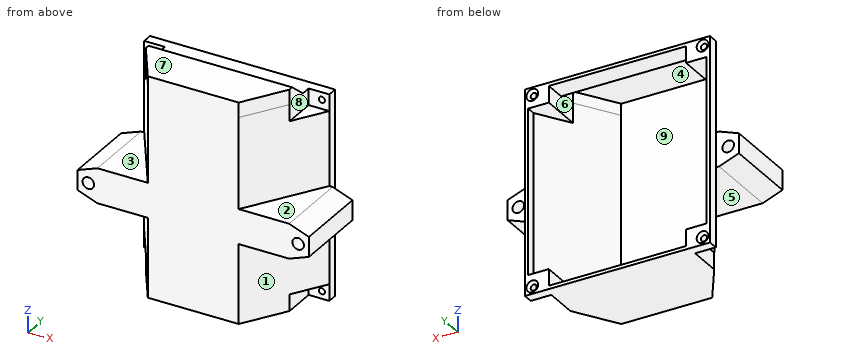
from build123d import *

# Parameters (mm, degrees)
MAIN_BODY_DEPTH                                   = 124
SKETCH38_W                                        = 112
SKETCH38_H                                        = 124
BOSS_EXTRUDE2_DEPTH                               = 6
SCREW_CUT_REACH                                   = 159.953
SKETCH22_W                                        = 12.496184963
SKETCH22_H                                        = 10
BOX_START                                         = -71.003815
BOX_EXTENSION_DEPTH                               = 87.00763
CUT_EXTRUDE1_DEPTH                                = 158.953315888
INNER_SHELL_T                                     = -2
ANGLE_SUPPORTS_DEPTH                              = 21
SCREW_START                                       = -45
SKETCH9_R                                         = 3.5
SKETCH9_W                                         = 2
SKETCH9_H                                         = 21
SCREW_SUPPORT_DEPTH                               = 45
SKETCH14_W                                        = 12.496184963
SKETCH14_H                                        = 10
BOX_SCREW_SUPPORT_DEPTH                           = 6
CSK_FOR_6_FLAT_HEAD_MACHINE_SCREW_100_D           = 3.6576
CSK_FOR_6_FLAT_HEAD_MACHINE_SCREW_100_CSINK_D     = 7.0866
CSK_FOR_6_FLAT_HEAD_MACHINE_SCREW_100_CSINK_ANGLE = 100
LPATTERN1_COUNT                                   = 2
LPATTERN1_PITCH                                   = 103
LPATTERN1_COUNT_DIR2                              = 2
LPATTERN1_PITCH_DIR2                              = 115


with BuildPart() as part:
    # Front face → Main Body (new body)
    with BuildSketch(Plane.XY):
        Polygon((-28.5, 45), (83.5, 45), (55, 0), (0, 0), align=None)
    extrude(amount=MAIN_BODY_DEPTH)

    # Sketch38 → Boss-Extrude2 (add)
    with BuildSketch(Plane(origin=(0, 45, 0), x_dir=(1, 0, 0), z_dir=(0, 1, 0))):
        with Locations((27.5, -62)):
            Rectangle(SKETCH38_W, SKETCH38_H)
    extrude(amount=BOSS_EXTRUDE2_DEPTH)

    # Sketch22 → Screw Cut (cut, up to next)
    with BuildSketch(Plane(origin=(0, 51, 0), x_dir=(1, 0, 0), z_dir=(0, 1, 0)), mode=Mode.PRIVATE) as screw_cut_sk1:
        with Locations((-22.251907519, -5)):
            Rectangle(SKETCH22_W, SKETCH22_H)
    screw_cut_tool1 = extrude(screw_cut_sk1.sketch, amount=-SCREW_CUT_REACH, mode=Mode.PRIVATE) & part.part
    # Sketch22 → Screw Cut (cut, up to next)
    with BuildSketch(Plane(origin=(0, 51, 0), x_dir=(1, 0, 0), z_dir=(0, 1, 0)), mode=Mode.PRIVATE) as screw_cut_sk2:
        with Locations((77.251907519, -5)):
            Rectangle(SKETCH22_W, SKETCH22_H)
    screw_cut_tool2 = extrude(screw_cut_sk2.sketch, amount=-SCREW_CUT_REACH, mode=Mode.PRIVATE) & part.part
    # Sketch22 → Screw Cut (cut, up to next)
    with BuildSketch(Plane(origin=(0, 51, 0), x_dir=(1, 0, 0), z_dir=(0, 1, 0)), mode=Mode.PRIVATE) as screw_cut_sk3:
        with Locations((77.251907519, -119)):
            Rectangle(SKETCH22_W, SKETCH22_H)
    screw_cut_tool3 = extrude(screw_cut_sk3.sketch, amount=-SCREW_CUT_REACH, mode=Mode.PRIVATE) & part.part
    # Sketch22 → Screw Cut (cut, up to next)
    with BuildSketch(Plane(origin=(0, 51, 0), x_dir=(1, 0, 0), z_dir=(0, 1, 0)), mode=Mode.PRIVATE) as screw_cut_sk4:
        with Locations((-22.251907519, -119)):
            Rectangle(SKETCH22_W, SKETCH22_H)
    screw_cut_tool4 = extrude(screw_cut_sk4.sketch, amount=-SCREW_CUT_REACH, mode=Mode.PRIVATE) & part.part
    add(screw_cut_tool1.solids().sort_by_distance((-22.251908, 51, 5))[0], mode=Mode.SUBTRACT)
    add(screw_cut_tool2.solids().sort_by_distance((77.251908, 51, 5))[0], mode=Mode.SUBTRACT)
    add(screw_cut_tool3.solids().sort_by_distance((77.251908, 51, 119))[0], mode=Mode.SUBTRACT)
    add(screw_cut_tool4.solids().sort_by_distance((-22.251908, 51, 119))[0], mode=Mode.SUBTRACT)

    # Sketch23 → Box Extension (add)
    with BuildSketch(Plane.ZY.offset(BOX_START)):
        Polygon((124, 0), (124, 39), (133.001495165, 28), (133.001495165, 0), align=None)
    extrude(amount=BOX_EXTENSION_DEPTH)

    # Sketch28 → Cut-Extrude1 (cut, through all)
    with BuildSketch(Plane(origin=(0, 0, 124), x_dir=(-1, 0, 0), z_dir=(0, 0, -1))):
        Polygon((-71.003815037, 0), (-55, 0), (-71.003815037, 25.269181637), align=None)
        Polygon((0, 0), (16.003815037, 0), (16.003815037, 25.269181637), align=None)
    extrude(amount=-CUT_EXTRUDE1_DEPTH, mode=Mode.SUBTRACT)

    # Inner Shell
    inner_shell_openings = [part.faces().sort_by_distance(p)[0] for p in [
        (27.5, 51, 62),
    ]]
    offset(amount=INNER_SHELL_T, openings=inner_shell_openings, kind=Kind.INTERSECTION)

    # Support → Angle supports (add)
    with BuildSketch(Plane(origin=(0, 0, 48), x_dir=(-1, 0, 0), z_dir=(0, 0, -1))):
        Polygon((0, 0), (28.5, 0), (28.5, 45), align=None)
        Polygon((-83.5, 45), (-55, 0), (-83.5, 0), align=None)
    extrude(amount=-ANGLE_SUPPORTS_DEPTH)

    # Sketch9 → Screw Support (add)
    # profile 1 of 4: a face of its own
    with BuildSketch(Plane.XZ.offset(SCREW_START)):
        Polygon((97.5, 64.5), (85.5, 69), (85.5, 48), (97.5, 52.5), align=None)
        with Locations(Location((91, 58.5, 0), (0, 0, 270))):
            Circle(SKETCH9_R, mode=Mode.SUBTRACT)
    # profile 2 of 4: a face of its own
    with BuildSketch(Plane.XZ.offset(SCREW_START)):
        with Locations((84.5, 58.5)):
            Rectangle(SKETCH9_W, SKETCH9_H)
    # profile 3 of 4: a face of its own
    with BuildSketch(Plane.XZ.offset(SCREW_START)):
        Polygon((-42.5, 52.5), (-30.5, 48), (-30.5, 69), (-42.5, 64.5), align=None)
        with Locations(Location((-36, 58.5, 0), (0, 0, 270))):
            Circle(SKETCH9_R, mode=Mode.SUBTRACT)
    # profile 4 of 4: a face of its own
    with BuildSketch(Plane.XZ.offset(SCREW_START)):
        with Locations((-29.5, 58.5)):
            Rectangle(SKETCH9_W, SKETCH9_H)
    extrude(amount=SCREW_SUPPORT_DEPTH)

    # Sketch14 → Box Screw support (add)
    with BuildSketch(Plane(origin=(0, 51, 0), x_dir=(1, 0, 0), z_dir=(0, 1, 0))):
        with Locations((-22.251907519, -5)):
            Rectangle(SKETCH14_W, SKETCH14_H)
        with Locations((77.251907519, -5)):
            Rectangle(SKETCH14_W, SKETCH14_H)
        with Locations((77.251907519, -119)):
            Rectangle(SKETCH14_W, SKETCH14_H)
        with Locations((-22.251907519, -119)):
            Rectangle(SKETCH14_W, SKETCH14_H)
    extrude(amount=-BOX_SCREW_SUPPORT_DEPTH)

    # CSK for #6 Flat Head Machine Screw (100)3 (through all)
    with Locations(Plane(origin=(-24, 51, 119.5), x_dir=(0, 0, 1), z_dir=(0, 1, 0))):
        with Locations((0, 0)):
            csk_for_6_flat_head_machine_screw_100 = CounterSinkHole(CSK_FOR_6_FLAT_HEAD_MACHINE_SCREW_100_D / 2, CSK_FOR_6_FLAT_HEAD_MACHINE_SCREW_100_CSINK_D / 2, counter_sink_angle=CSK_FOR_6_FLAT_HEAD_MACHINE_SCREW_100_CSINK_ANGLE)

    # LPattern1: CSK for _6 Flat Head Machine Screw _100 2 × 2
    with Locations(*[(i * LPATTERN1_PITCH, 0, -j * LPATTERN1_PITCH_DIR2) for i in range(LPATTERN1_COUNT) for j in range(LPATTERN1_COUNT_DIR2) if (i, j) != (0, 0)]):
        add(csk_for_6_flat_head_machine_screw_100, mode=Mode.SUBTRACT)


solid = part.part
Build history of the part. All positions in model axes, mm. Face numbers are marked on the shaded views. A direction names the side the tool comes from. Round coordinates to 2 decimals unless told otherwise and drop trailing zeros. Loops run counter-clockwise (first coordinate to the right, second up) from the corner with the lowest first, then second, coordinate; pieces in that order, holes last. Notation, with made-up numbers: (37.5, 55) -> (69.5, 55) arc R22 cw to (69.5, 76) -> close; hole circle Ø6 at (79.25, 9). An arc over 180 degrees is marked (long way). Answer in a Markdown table with one row per item.
Item 1: Saw through at D-D (y = 13). Write the cut outline in (x, z).
Answers below:
| item | result |
|---|---|
| outline | (-42.5, 52.5) -> (-30.5, 48) -> (-8.23, 48) -> (-8.23, 0) -> (63.23, 0) -> (63.23, 48) -> (85.5, 48) -> (97.5, 52.5) -> (97.5, 64.5) -> (85.5, 69) -> (63.23, 69) -> (63.23, 133) -> (-8.23, 133) -> (-8.23, 69) -> (-30.5, 69) -> (-42.5, 64.5) -> close; hole circle Ø7 at (-36, 58.5); hole (-5.87, 2) -> (60.87, 2) -> (60.87, 131) -> (-5.87, 131) -> close; hole circle Ø7 at (91, 58.5) |
Item 2: Mould opens along Z. For the marked faces 6, 7, 8 and 9 say: +Z half, -Z half, draft (parallel to the pull), parting line (faces both ways), or undercut.
Answers below:
| item | result |
|---|---|
| face 6 | undercut |
| face 7 | +Z half |
| face 8 | draft |
| face 9 | undercut |
Item 3: Saw through at C-C (x = -24). Write the cut outline in (y, z), and give its area (3 significant figures).
Answers below:
| item | result |
|---|---|
| outline | (0, 48) -> (37.89, 48) -> (37.89, 10) -> (45, 10) -> (45, 6.33) -> (49.56, 6.33) -> (51, 8.04) -> (51, 12) -> (41.63, 12) -> (41.63, 112) -> (51, 112) -> (51, 115.96) -> (49.56, 117.67) -> (45, 117.67) -> (45, 114) -> (37.89, 114) -> (37.89, 69) -> (0, 69) -> close; (45, 0) -> (51, 0) -> (51, 0.96) -> (49.56, 2.67) -> (45, 2.67) -> close; (45, 121.33) -> (49.56, 121.33) -> (51, 123.04) -> (51, 124) -> (45, 124) -> close |
| area | 1,290 mm² |
Item 4: Saw through at A-A (z = 58.5). Write the cut outline in (x, y), and give its area (3 significant figures).
Answers below:
| item | result |
|---|---|
| outline | (-42.5, 0) -> (-39.5, 0) -> (-39.5, 45) -> (-42.5, 45) -> close; (-32.5, 0) -> (87.5, 0) -> (87.5, 45) -> (83.5, 45) -> (83.5, 51) -> (81.5, 51) -> (81.5, 45.58) -> (53.9, 2) -> (1.1, 2) -> (-26.5, 45.58) -> (-26.5, 51) -> (-28.5, 51) -> (-28.5, 45) -> (-32.5, 45) -> close; (94.5, 0) -> (97.5, 0) -> (97.5, 45) -> (94.5, 45) -> close |
| area | 2,250 mm² |
Item 5: Saw through at B-B (z = 101.5). Write the cut outline in (x, y), and give its area (3 significant figures).
Answers below:
| item | result |
|---|---|
| outline | (-28.5, 45) -> (0, 0) -> (55, 0) -> (83.5, 45) -> (83.5, 51) -> (81.5, 51) -> (81.5, 45.58) -> (53.9, 2) -> (1.1, 2) -> (-26.5, 45.58) -> (-26.5, 51) -> (-28.5, 51) -> close |
| area | 340 mm² |
Item 6: Which spindle directions (+Z, -Z, +X, -X, +Y, -Y) get a long thin tool onto all of the face, cutting with end or side? Do the marked faces 1, 2, 3, 4 and 5. Say none if no direction does.
Answers below:
| item | result |
|---|---|
| face 1 | -Z, +X, -Y |
| face 2 | +Z, +X, -Y |
| face 3 | +Z, -X, -Y |
| face 4 | none |
| face 5 | -Z, -X, -Y |
Item 7: Drill centre lines: L1, parallel to Z at x = -24, y = 46; L2, parallel to X at y = 46.85, z = 119.5; L3, parallel to Z at x = 45, y = 6. Where is each one in solid material? Low to high. Write a range as [from, to].
Answers below:
| item | result |
|---|---|
| L1 | z = [0, 2.67], [6.33, 12], [112, 117.67], [121.33, 124] |
| L2 | x = [-28.5, -25.83], [-22.17, -14], [69, 77.17], [80.83, 83.5] |
| L3 | z = [0, 2], [131, 133] |
Item 8: Pin check, flat tips, straight feed: pin 1 (5 mm diameter, centred on x = -11.5, y = 40, fed in from +Z); pin 2 (5 mm diameter, centred on x = 10.5, z = 37, fed in from +Y); pin 3 (6.5 mm diameter, centred on x = -36, z = 58.5, fed in from -Y); pin 4 (9.5 mm diameter, centred on y = 32.5, z = 123, fed in from +X). Stop position of each tip, or through.
Answers below:
| item | result |
|---|---|
| pin 1 | stops at z = 125.23 |
| pin 2 | stops at y = 2 |
| pin 3 | passes through |
| pin 4 | stops at x = 71 |
